```python
from build123d import *

# Parameters (mm, degrees)
F0_W     = 35
F0_H     = 20
F1_DEPTH = 10
F2_R     = 0.75
F2_R_2   = 2.5
F3_DEPTH = 6.5
F4_DEPTH = 2
F5_DEPTH = 25
F6_SIZE2 = 6
F6_SIZE  = 6
F7_SIZE  = 1
F8_SIZE2 = 2.1838214056
F8_SIZE  = 6


with BuildPart() as f1:
    # F0 (on Top) → F1 (new body)
    with BuildSketch(Plane.XY):
        with Locations((17.5, 10)):
            Rectangle(F0_W, F0_H)
    extrude(amount=F1_DEPTH)

    # F2 (on face) → F3 (cut)
    with BuildSketch(Plane.XY.offset(10)):
        Polygon((35, 18.2), (0, 18.2), (0, 0), (11.5, 0), (11.5, 6), (23.5, 6), (23.5, 0), (35, 0), align=None)
        with Locations((7.5, 12.7)):
            Circle(F2_R, mode=Mode.SUBTRACT)
        with Locations((13.75, 12.7)):
            Circle(F2_R_2, mode=Mode.SUBTRACT)
        with Locations((21.25, 12.7)):
            Circle(F2_R_2, mode=Mode.SUBTRACT)
        with Locations((27.5, 12.7)):
            Circle(F2_R, mode=Mode.SUBTRACT)
    extrude(amount=-F3_DEPTH, mode=Mode.SUBTRACT)

    # F4 (cut): faces of the model
    f4_faces = [f1.faces().sort_by_distance(p)[0] for p in [
        (7.5, 12.7, 10),
        (17.5, 3, 10),
        (27.5, 12.7, 10),
    ]]
    extrude(f4_faces, amount=-F4_DEPTH, mode=Mode.SUBTRACT)

    # F5 (cut): faces of the model
    f5_faces = [f1.faces().sort_by_distance(p)[0] for p in [
        (13.75, 12.7, 10),
        (21.25, 12.7, 10),
    ]]
    extrude(f5_faces, amount=-F5_DEPTH, mode=Mode.SUBTRACT)

    # F6
    f6_edges = [f1.edges().sort_by_distance(p)[0] for p in [
        (35, 0, 1.75),
        (35, 20, 5),
        (0, 0, 1.75),
        (0, 20, 5),
    ]]
    chamfer(f6_edges, length=F6_SIZE, length2=F6_SIZE2)

    # F7
    f7_edges = [f1.edges().sort_by_distance(p)[0] for p in [
        (17.5, 20, 0),
        (32, 17, 0),
        (3, 17, 0),
        (17.5, 18.2, 10),
        (17.5, 6, 8),
        (23.5, 3, 8),
        (11.5, 3, 8),
        (35, 10, 0),
        (0, 10, 0),
        (18.75, 12.7, 0),
        (11.25, 12.7, 0),
        (3, 3, 0),
        (32, 3, 0),
    ]]
    chamfer(f7_edges, length=F7_SIZE)

    # F8
    f8_edges = [f1.edges().sort_by_distance(p)[0] for p in [
        (17.5, 0, 0),
    ]]
    f8_side = f1.faces().sort_by_distance((17.5, 0, 3.355675))[0]
    chamfer(f8_edges, length=F8_SIZE, length2=F8_SIZE2, reference=f8_side)


solid = f1.part
```
Geometry check sheet. Reference: the model listing, model coordinates, mm. A direction names the side the tool comes from. Round coordinates to 2 decimals unless told otherwise and drop trailing zeros. Order: outer loops, then holes, each group sorted by start corner. A loop starts at its lowest first (then second) coordinate and runs counter-clockwise, first axis right, second up. Notation, with made-up numbers: (-7.5, -22) - (32.5, -22) arc R19 cw to (32.5, 6) - close; hole circle Ø6 at (89, 28.25). An arc over 180 degrees is marked (long way). Use a Markdown table: item, result. Add a question column.
1) Section check B-B (y = 12.7). Record the cut outline in (x, z), then the cut area to 3 significant figures.
2) Section check A-A (x = 21.25). Record the cut outline in (y, z), then the cut area to 3 significant figures.
3) Set-up check for faces 5 (the flat face through (23, 3, 7.5)), 6 (the flat face through (17.3, 19.6, 10)), 7 (the flat face through (11.5, 3, 5)), 8 (the flat face through (7, 13, 8)), 9 (the flat face through (17.4, 5.5, 7.5)): record each of +Z, -Z, +X, -X, +Y, -Y from which the full face is reachable in a straight line by a thin tool's end or side.
4) Gauge pin test, flat ends, axial feed: P1, Ø2, axis at x = 20.5, y = 6.5, coming from the +Z side; P2, Ø4, axis at y = 3.5, z = 5, coming from the +X side; P3, Ø2, axis at x = 26, y = 11.5, coming from the +Z side. Record the tip position at first contact, or that the pin passes through.
5) Mould release check, pull along Y, two halves, no side actions. Record for faces 1 (the cylindrical face through (11.252, 12.81, 2.268)), 2 (the flat face through (17, 20, 5)), 3 (the cylindrical face through (6.905, 12.244, 5.781)), 4 (the flat face through (27, 13, 8)): released by +Y, released by -Y, zero draft, split by the parting line, or undercut.
6) Section check D-D (x = 9). Record the cut outline in (y, z), then the cut area to 3 significant figures.
7) Section check C-C (z = 1.5). Record the cut outline in (x, y), then the cut area to 3 significant figures.
8) Thickness scan on line 1 along Z through (x, y) = (9, 16.5); line 2 along Y through (x, z) = (13.75, 1.8); line 3 along Y through (x, z) = (21.25, 2.45). Record the ranges inside material, lowest first.
Established:
| question | item | result |
|---|---|---|
| 1 | outline | (0, 1) - (1, 0) - (10.25, 0) - (11.25, 1) - (11.25, 3.5) - (8.25, 3.5) - (8.25, 8) - (6.75, 8) - (6.75, 3.5) - (0, 3.5) - close; (16.25, 1) - (17.25, 0) - (17.75, 0) - (18.75, 1) - (18.75, 3.5) - (16.25, 3.5) - close; (23.75, 1) - (24.75, 0) - (34, 0) - (35, 1) - (35, 3.5) - (28.25, 3.5) - (28.25, 8) - (26.75, 8) - (26.75, 3.5) - (23.75, 3.5) - close |
| 1 | area | 98.0 mm2 |
| 2 | outline | (0, 6) - (2.18, 0) - (9.2, 0) - (10.2, 1) - (10.2, 3.5) - (6, 3.5) - (6, 7) - (5, 8) - (0, 8) - close; (15.2, 1) - (16.2, 0) - (19, 0) - (20, 1) - (20, 10) - (19.2, 10) - (18.2, 9) - (18.2, 3.5) - (15.2, 3.5) - close |
| 2 | area | 82.1 mm2 |
| 3 | face 5 | +Z, +X, -Y |
| 3 | face 6 | +Z, +X, -X, +Y, -Y |
| 3 | face 7 | +Z, -X, -Y |
| 3 | face 8 | +Z, +X, -X, -Y |
| 3 | face 9 | +Z, +X, -X |
| 4 | P1 | z = 7.5 |
| 4 | P2 | x = 33.82 |
| 4 | P3 | z = 3.5 |
| 5 | face 1 | undercut |
| 5 | face 2 | released by +Y |
| 5 | face 3 | undercut |
| 5 | face 4 | zero draft |
| 6 | outline | (0.91, 3.5) - (2.18, 0) - (19, 0) - (20, 1) - (20, 10) - (19.2, 10) - (18.2, 9) - (18.2, 3.5) - close |
| 6 | area | 75.3 mm2 |
| 7 | outline | (0, 6) - (4.36, 1.64) - (30.64, 1.64) - (35, 6) - (35, 14) - (29, 20) - (6, 20) - (0, 14) - close; hole circle Ø5 at (13.75, 12.7); hole circle Ø5 at (21.25, 12.7) |
| 7 | area | 548 mm2 |
| 8 | line 1 | 0 to 3.5 |
| 8 | line 2 | 1.53 to 10.2, 15.2 to 20 |
| 8 | line 3 | 1.29 to 10.2, 15.2 to 20 |
